The listing builds one solid part. Answer for the finished solid, in the listing's coordinates (mm). Face numbers are marked on the shaded views. A direction names the side the tool comes from. Coordinates: 2 decimals unless noted, no trailing zeros. Order: outer loops, then holes, each group sorted by start corner. A loop starts at its lowest first (then second) coordinate and runs counter-clockwise, first axis right, second up. Notation, with made-up numbers: (27.5, 15.25) -> (68.5, 15.25) arc R14 ccw to (68.5, 35.25) -> close; hole circle Ø3 at (55.5, 49). An arc over 180 degrees is marked (long way). Answer in a Markdown table with one row per item.
```python
from build123d import *

# Parameters (mm, degrees)
BOSS_EXTRUDE1_DEPTH = 3.175
SKETCH2_R           = 7.95
BOSS_EXTRUDE2_DEPTH = 11.825
SKETCH3_R           = 5.4
BOSS_EXTRUDE3_DEPTH = 9.3
SKETCH4_W           = 0.4
SKETCH4_H           = 1.8
BOSS_EXTRUDE4_DEPTH = 5.4
FILLET1_R           = 0.889
CUT_EXTRUDE1_DEPTH  = 31.396309398
SKETCH6_R           = 8.589918765
BOSS_EXTRUDE5_DEPTH = 1.7
BOSS_EXTRUDE5_TAPER = 50
SKETCH8_R           = 6.563937658
SKETCH8_R_2         = 5.1943
CUT_EXTRUDE2_DEPTH  = 0.0254


with BuildPart() as part:
    # Sketch1 → Boss-Extrude1 (new body)
    with BuildSketch(Plane(origin=(0, 0, 0), x_dir=(1, 0, 0), z_dir=(0, 1, 0))):
        Polygon((9, 5.196152423), (0, 10.392304845), (-9, 5.196152423), (-9, -5.196152423), (0, -10.392304845), (9, -5.196152423), align=None)
    extrude(amount=BOSS_EXTRUDE1_DEPTH)

    # Sketch2 → Boss-Extrude2 (add)
    with BuildSketch(Plane.XZ):
        with Locations(Location((0, 0, 0), (0, 0, 90))):
            Circle(SKETCH2_R)
    extrude(amount=BOSS_EXTRUDE2_DEPTH)

    # Sketch3 → Boss-Extrude3 (add)
    with BuildSketch(Plane.XZ.offset(11.825)):
        with Locations(Location((0, 0, 0), (0, 0, 90))):
            Circle(SKETCH3_R)
    extrude(amount=BOSS_EXTRUDE3_DEPTH)

    # Sketch4 → Boss-Extrude4 (add)
    with BuildSketch(Plane.XZ.offset(21.125)):
        with Locations((-1.4, 2.5)):
            Rectangle(SKETCH4_W, SKETCH4_H)
        with Locations((-1.4, -2.5)):
            Rectangle(SKETCH4_W, SKETCH4_H)
        with Locations((1.4, 0)):
            Rectangle(SKETCH4_W, SKETCH4_H)
    extrude(amount=BOSS_EXTRUDE4_DEPTH)

    # Fillet1
    fillet1_edges = [part.edges().sort_by_distance(p)[0] for p in [
        (-1.4, -26.525, 1.6),
        (-1.4, -26.525, 3.4),
        (-1.4, -26.525, -3.4),
        (-1.4, -26.525, -1.6),
        (1.4, -26.525, -0.9),
        (1.4, -26.525, 0.9),
    ]]
    fillet(fillet1_edges, radius=FILLET1_R)

    # Sketch5 → Cut-Extrude1 (cut, through all)
    with BuildSketch(Plane(origin=(1.6, 0, 0), x_dir=(0, 0, -1), z_dir=(1, 0, 0))):
        with BuildLine():
            Line((-0.37, -25.636), (-0.37, -24.366))
            ThreePointArc((-0.37, -24.366), (0.011, -23.985), (0.392, -24.366))
            Line((0.392, -24.366), (0.392, -25.636))
            ThreePointArc((0.392, -25.636), (0.011, -26.017), (-0.37, -25.636))
        make_face()
        with BuildLine():
            Line((-2.87, -25.636), (-2.87, -24.366))
            ThreePointArc((-2.87, -24.366), (-2.489, -23.985), (-2.108, -24.366))
            Line((-2.108, -24.366), (-2.108, -25.636))
            ThreePointArc((-2.108, -25.636), (-2.489, -26.017), (-2.87, -25.636))
        make_face()
        with BuildLine():
            Line((2.108, -25.636), (2.108, -24.366))
            ThreePointArc((2.108, -24.366), (2.489, -23.985), (2.87, -24.366))
            Line((2.87, -24.366), (2.87, -25.636))
            ThreePointArc((2.87, -25.636), (2.489, -26.017), (2.108, -25.636))
        make_face()
    extrude(amount=-CUT_EXTRUDE1_DEPTH, mode=Mode.SUBTRACT)

    # Sketch6 → Boss-Extrude5 (add)
    with BuildSketch(Plane(origin=(0, 3.175, 0), x_dir=(1, 0, 0), z_dir=(0, 1, 0))):
        Circle(SKETCH6_R)
    extrude(amount=BOSS_EXTRUDE5_DEPTH, taper=BOSS_EXTRUDE5_TAPER)

    # Sketch7 → Cut-Revolve1 (revolve, cut)
    with BuildSketch(Plane(origin=(0, 0, 0), x_dir=(0, 0, -1), z_dir=(1, 0, 0))):
        with BuildLine():
            Line((7.885247447, 3.175), (10.392304845, 3.175))
            Line((10.392304845, 3.175), (10.392304845, 2.354871392))
            ThreePointArc((10.392304845, 2.354871392), (9.18924806, 2.919223674), (7.885247447, 3.175))
        make_face()
    cut_revolve1 = revolve(axis=Axis((0, 0, 0), (0, 1, 0)), mode=Mode.SUBTRACT)

    # Mirror1: Cut-Revolve1 across plane
    add(cut_revolve1.mirror(Plane(origin=(0, 1.5875, 0), x_dir=(0, 0, 1), z_dir=(0, -1, 0))), mode=Mode.SUBTRACT)

    # Sketch8 → Cut-Extrude2 (cut)
    with BuildSketch(Plane(origin=(0, 4.875, 0), x_dir=(1, 0, 0), z_dir=(0, 1, 0))):
        with Locations(Location((0, 0, 0), (0, 0, 270))):
            Circle(SKETCH8_R)
        with Locations(Location((0, 0, 0), (0, 0, 270))):
            Circle(SKETCH8_R_2, mode=Mode.SUBTRACT)
    extrude(amount=-CUT_EXTRUDE2_DEPTH, mode=Mode.SUBTRACT)


solid = part.part
```
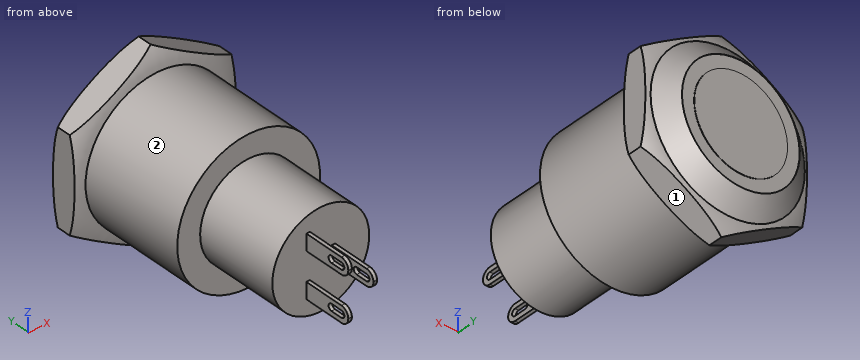
(1) Flat-ended cylindrical pins translate along their axes: pin 1 (0.9 mm diameter, centred on y = -24, z = -3, fed in from -X); pin 2 (1.4 mm diameter, centred on y = -23, z = -2, fed in from +X); pin 3 (4 mm diameter, centred on y = -17.5, z = 3.5, fed in from -X). Find the tip coordinate at first contact, or state that the pin passes through.
Check values:
| item | result |
|---|---|
| pin 1 | x = -1.6 |
| pin 2 | x = -1.2 |
| pin 3 | x = -5.19 |
(2) A cutting plane is placed at A-A, the plane y = -15.5. Determine the outline of the cut face in (x, z), then the cut area to 3 significant figures.
Check values:
| item | result |
|---|---|
| outline | circle Ø10.8 at (0, 0) |
| area | 91.6 mm² |
(3) Find the intervals of material crossed by line 1 along Y through (x, z) = (-3, 5.5) (3 decimals); line 2 along Y through (x, z) = (-0.25, 5) (3 decimals); line 3 along X through (y, z) = (-21, 0.5), in increasing order. Write a range as from..to.
Check values:
| item | result |
|---|---|
| line 1 | -11.825..4.85 |
| line 2 | -21.125..4.875 |
| line 3 | -5.38..5.38 |
(4) A cutting plane is placed at B-B, the plane y = -4.5. Determine the outline of the cut face in (x, z).
Check values:
| item | result |
|---|---|
| outline | circle Ø15.9 at (0, 0) |
(5) Which of the six approach directions +Z, -Z, +X, -X, +Y, -Y give full straight-line access (tool end or side, diameter ignored) to the marked faces 1 and 2?
Check values:
| item | result |
|---|---|
| face 1 | -Z, +X, +Y, -Y |
| face 2 | -Y |
